Here's how the part is built. I have some questions about the finished solid (model axes, mm). Face numbers are marked on the shaded views. Round coordinates to 2 decimals unless told otherwise and drop trailing zeros. Order: outer loops, then holes, each group sorted by start corner. A loop starts at its lowest first (then second) coordinate and runs counter-clockwise, first axis right, second up. Notation, with made-up numbers: (72.5, 53) -> (84.5, 53) arc R23 cw to (84.5, 64) -> close; hole circle Ø4 at (-26.75, 6). An arc over 180 degrees is marked (long way). Answer in a Markdown table with one row per item.
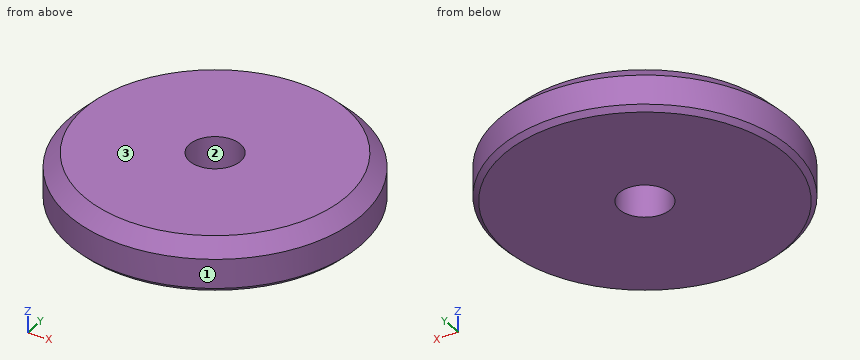
```python
from build123d import *

# Parameters (mm, degrees)
SKETCH_2_R      = 30
SKETCH_2_R_2    = 5.25
EXTRUDE_1_DEPTH = 10
CHAMFER_1_SIZE  = 3
CHAMFER_2_SIZE  = 1


with BuildPart() as part:
    # Эскиз2 → Бобышка-Вытянуть1 (new body)
    with BuildSketch(Plane.XY):
        Circle(SKETCH_2_R)
        Circle(SKETCH_2_R_2, mode=Mode.SUBTRACT)
    extrude(amount=EXTRUDE_1_DEPTH)

    # Фаска1
    chamfer_1_edges = [part.edges().sort_by_distance(p)[0] for p in [
        (-30, 0, 10),
    ]]
    chamfer(chamfer_1_edges, length=CHAMFER_1_SIZE)

    # Фаска2
    chamfer_2_edges = [part.edges().sort_by_distance(p)[0] for p in [
        (-30, 0, 0),
    ]]
    chamfer(chamfer_2_edges, length=CHAMFER_2_SIZE)


solid = part.part
```
1. Suppose I cut it at A-A on y = 0. Write out the boundary of the cut face in (x, z).
Numbers:
| item | result |
|---|---|
| outline | (-30, 1) -> (-29, 0) -> (-5.25, 0) -> (-5.25, 10) -> (-27, 10) -> (-30, 7) -> close; (5.25, 0) -> (29, 0) -> (30, 1) -> (30, 7) -> (27, 10) -> (5.25, 10) -> close |
2. Please list where these lines run through material, in increasing order: line 1 along Y through (x, z) = (0, 2.5); line 2 along X through (y, z) = (4, 6.25); line 3 along Y through (x, z) = (3, 1.5).
Numbers:
| item | result |
|---|---|
| line 1 | y = -30 to -5.25, 5.25 to 30 |
| line 2 | x = -29.73 to -3.4, 3.4 to 29.73 |
| line 3 | y = -29.85 to -4.31, 4.31 to 29.85 |
3. For pin 1 Ø6 at (y, z) = (-2, 6) entering from +X; pin 2 Ø2 at (x, z) = (-6.5, 3) entering from -Y; pin 3 Ø9.5 at (x, y) = (0, 0) entering from -Z; pin 4 Ø5 at (x, z) = (8.5, 3) entering from +Y, each with a flat end and sliding along its axis, tell me the tip position at first contact or that it passes through.
Numbers:
| item | result |
|---|---|
| pin 1 | stops at x = 30 |
| pin 2 | stops at y = -29.49 |
| pin 3 | passes through |
| pin 4 | stops at y = 29.39 |
4. We'd pull the mould along Y, two halves only. Please class the marked faces 1, 2 and 3: released by +Y, released by -Y, zero draft, split by the parting line, or undercut.
Numbers:
| item | result |
|---|---|
| face 1 | split by the parting line |
| face 2 | undercut |
| face 3 | zero draft |
5. Suppose I cut it at C-C on z = 4. Write out the boundary of the cut face in (x, y), then the cut area to 3 significant figures.
Numbers:
| item | result |
|---|---|
| outline | circle Ø60 at (0, 0); hole circle Ø10.5 at (0, 0) |
| area | 2,740 mm2 |
